Part model, mm, in its own coordinate system. A direction names the side the tool comes from. Round coordinates to 2 decimals unless told otherwise and drop trailing zeros. Loops run counter-clockwise (first coordinate to the right, second up) from the corner with the lowest first, then second, coordinate; pieces in that order, holes last. Notation, with made-up numbers: (13, 44.5) - (50, 44.5) arc R12 ccw to (50, 64.5) - close; hole circle Ø9 at (8, 20.25). An arc over 180 degrees is marked (long way). Put each result on its own line as item: value.
from build123d import *

# Parameters (mm, degrees)
F0_R      = 29.21
F1_DEPTH  = 304.165
F2_W      = 34.29
F2_H      = 17.78
F3_DEPTH  = 38.1
F4_R      = 17.14499
F5_R      = 11.43
F6_DEPTH  = 3.81
F7_R      = 11.43
F8_DEPTH  = 3.81
F9_R      = 6.35
F10_DEPTH = 38.1


# Not quite as in the source:
# - a fillet or chamfer is up to 0.001 mm smaller than in the source, because OpenCascade refuses the exact size


with BuildPart() as f1:
    # F0 (on Top) → F1 (new body)
    with BuildSketch(Plane.XY):
        Circle(F0_R)
    extrude(amount=F1_DEPTH)

    # F2 (on face) → F3 (join)
    with BuildSketch(Plane.XY.offset(304.165)):
        Rectangle(F2_W, F2_H)
    extrude(amount=F3_DEPTH)

    # F4 (radius 17.145 in the source; OpenCascade refuses exactly that, so slightly less here)
    f4_edges = [f1.edges().sort_by_distance(p)[0] for p in [
        (17.145, 0, 342.265),
        (-17.145, 0, 342.265),
    ]]
    fillet(f4_edges, radius=F4_R)

    # F5 (on face) → F6 (join)
    with BuildSketch(Plane(origin=(0, 8.89, 0), x_dir=(-1, 0, 0), z_dir=(0, 1, 0))):
        with Locations((0, 325.12)):
            Circle(F5_R)
    extrude(amount=F6_DEPTH)

    # F7 (on face) → F8 (join)
    with BuildSketch(Plane.XZ.offset(8.89)):
        with Locations((0, 325.12)):
            Circle(F7_R)
    extrude(amount=F8_DEPTH)

    # F9 (on face) → F10 (cut)
    with BuildSketch(Plane.XZ.offset(12.7)):
        with Locations((0, 325.12)):
            Circle(F9_R)
    extrude(amount=-F10_DEPTH, mode=Mode.SUBTRACT)


solid = f1.part
1. Band-saw the part on C-C (z = 187.5). List the corners of the cut face in (x, y).
A:
outline: circle Ø58.42 at (0, 0)
2. Band-saw the part on D-D (y = 21.5). List the corners of the cut face in (x, z) (3 decimals).
A:
outline: (-19.773, 0) - (19.773, 0) - (19.773, 304.165) - (-19.773, 304.165) - close
3. Two-plate mould, pull along X, no slides. Class faces 6 (the flat face through (-17.145, 0, 314)), 7 (the cylindrical face through (-0.827, -0.178, 331.416)), 8 (the flat face through (17.145, 0, 314)), 9 (the flat face through (-8, -8.89, 314)): pulls with the +X half, pulls with the -X half, needs draft (parallel to the pull), parting line crosses it, or undercut.
A:
face 6: pulls with the -X half
face 7: undercut
face 8: pulls with the +X half
face 9: needs draft
4. Tool access for faces 1 (the cylindrical face through (6.14, -10.77, 334.76)), 2 (the flat face through (0, 0, 0)), 3 (the flat face through (5, -12.7, 320)), 4 (the cylindrical face through (-6.14, 10.77, 334.76)), 5 (the flat face through (-5, 12.7, 320)): list every direction of +Z, -Z, +X, -X, +Y, -Y with a clear straight run to the whole face (end or side of a thin tool).
A:
face 1: -Y
face 2: -Z, +X, -X, +Y, -Y
face 3: +Z, +X, -X, -Y
face 4: +Y
face 5: +Z, +X, -X, +Y
5. Pin check, flat tips, straight feed: P1, Ø6, axis at y = 18, z = 200.5, coming from the +X side; P2, Ø10.5, axis at x = 4.5, z = 314, coming from the -Y side; P3, Ø20.5, axis at x = 0, z = 325.12, coming from the +Y side; P4, Ø19.5, axis at y = 2, z = 312.5, coming from the +X side. Stop position of each tip, or through.
A:
P1: stops at x = 25.06
P2: stops at y = -12.7
P3: stops at y = 12.7
P4: stops at x = 29.21
6. Probe line 1 along X through (y, z) = (-7, 325) (3 decimals); line 2 along Z through (x, y) = (-4.5, -2); line 3 along Z through (x, y) = (-21, -19.5) (3 decimals). List the from-to ranges inside material, lowest first. Write a range as [from, to].
A:
line 1: x = [-17.145, -6.349], [6.349, 17.145]
line 2: z = [0, 320.64], [329.6, 341.66]
line 3: z = [0, 304.165]
7. Band-saw the part on B-B (x = 3). List the corners of the cut face in (y, z) (1 decimal), plus the area to 3 significant figures.
A:
outline: (-29.1, 0) - (29.1, 0) - (29.1, 304.2) - (8.9, 304.2) - (8.9, 314.1) - (12.7, 314.1) - (12.7, 319.5) - (-12.7, 319.5) - (-12.7, 314.1) - (-8.9, 314.1) - (-8.9, 304.2) - (-29.1, 304.2) - close; (-12.7, 330.7) - (12.7, 330.7) - (12.7, 336.1) - (8.9, 336.1) - (8.9, 342) - (-8.9, 342) - (-8.9, 336.1) - (-12.7, 336.1) - close
area: 18,200 mm²
